Check sheet for the modelled part. Datum: model origin and axes. Units: mm. A direction names the side the tool comes from. Give positions to 0.01 mm unless a question says otherwise; leave off trailing zeros.
from build123d import *

# Parameters (mm, degrees)
SKETCH_4_W          = 150
SKETCH_4_H          = 100
EXTRUDE_1_DEPTH     = 19
EXTRUDE_1_TAPER     = 15
SHELL_1_T           = -2
SKETCH_13_R         = 1.5
CUT_EXTRUDE_3_DEPTH = 92.727858519
CUT_EXTRUDE_4_REACH = 94.119
SKETCH_15_R         = 3.5
SKETCH_16_R         = 2.5
CUT_EXTRUDE_5_DEPTH = 153.623831333


with BuildPart() as part:
    # 草图4 → 凸台-拉伸1 (new body)
    with BuildSketch(Plane(origin=(0, 0, 0), x_dir=(1, 0, 0), z_dir=(0, 1, 0))):
        Rectangle(SKETCH_4_W, SKETCH_4_H)
    extrude(amount=EXTRUDE_1_DEPTH, taper=EXTRUDE_1_TAPER)

    # 抽壳1
    shell_1_openings = [part.faces().sort_by_distance(p)[0] for p in [
        (0, 0, 0),
    ]]
    offset(amount=SHELL_1_T, openings=shell_1_openings, kind=Kind.INTERSECTION)

    # 草图13 → 切除-拉伸3 (cut, through all)
    with BuildSketch(Plane.XZ.offset(-17)):
        with Locations(Location((11, 15, 0), (0, 0, 270))):
            Circle(SKETCH_13_R)
        with Locations(Location((-11, 15, 0), (0, 0, 90))):
            Circle(SKETCH_13_R)
        with Locations(Location((11, -15, 0), (0, 0, 90))):
            Circle(SKETCH_13_R)
        with Locations(Location((-11, -15, 0), (0, 0, 270))):
            Circle(SKETCH_13_R)
    extrude(amount=-CUT_EXTRUDE_3_DEPTH, mode=Mode.SUBTRACT)

    # 切除-拉伸4: up to this plane
    cut_extrude_4_end = Plane(origin=(-75, 0, 50), z_dir=(-0.9659258262890681, 0.2588190451025214, 0))
    # 草图15 → 切除-拉伸4 (cut, up to the surface)
    with BuildSketch(Plane(origin=(0, 0, 0), x_dir=(0, 0, -1), z_dir=(1, 0, 0)), mode=Mode.PRIVATE) as cut_extrude_4_sk1:
        with Locations(Location((-35, 9.5, 0), (0, 0, 90))):
            Circle(SKETCH_15_R)
    cut_extrude_4_tool1 = split(extrude(cut_extrude_4_sk1.sketch, amount=-CUT_EXTRUDE_4_REACH, mode=Mode.PRIVATE), bisect_by=cut_extrude_4_end, keep=Keep.BOTH, mode=Mode.PRIVATE)
    add(cut_extrude_4_tool1.solids().sort_by_distance((0, 9.5, 35))[0], mode=Mode.SUBTRACT)
    # 草图15 → 切除-拉伸4 (cut, up to the surface)
    with BuildSketch(Plane(origin=(0, 0, 0), x_dir=(0, 0, -1), z_dir=(1, 0, 0)), mode=Mode.PRIVATE) as cut_extrude_4_sk2:
        with Locations(Location((35, 9.5, 0), (0, 0, 90))):
            Circle(SKETCH_15_R)
    cut_extrude_4_tool2 = split(extrude(cut_extrude_4_sk2.sketch, amount=-CUT_EXTRUDE_4_REACH, mode=Mode.PRIVATE), bisect_by=cut_extrude_4_end, keep=Keep.BOTH, mode=Mode.PRIVATE)
    add(cut_extrude_4_tool2.solids().sort_by_distance((0, 9.5, -35))[0], mode=Mode.SUBTRACT)

    # 草图16 → 切除-拉伸5 (cut, through all)
    with BuildSketch(Plane(origin=(68.044100989, 18.23236191, 0), x_dir=(0, 0, 1), z_dir=(-0.9659258262890681, -0.2588190451025214, 0))):
        with Locations(Location((0, -11.275834931, 0), (0, 0, 270))):
            Circle(SKETCH_16_R)
    extrude(amount=-CUT_EXTRUDE_5_DEPTH, mode=Mode.SUBTRACT)


solid = part.part
1) Depth check by flat-ended pin: pin 1 Ø4 at (x, z) = (60, 25.5) entering from -Y; pin 2 Ø5 at (y, z) = (6.5, 0.5) entering from -X; pin 3 Ø8 at (y, z) = (9.5, 35) entering from -X. Enter the tip coordinate at first touch or a pass-through.
Recorded:
pin 1: stops at y = 17
pin 2: stops at x = -73.93
pin 3: stops at x = -73.53
2) Set-up check for faces 4 (the face through (-2, 19, 0)), 5 (the face through (-2, 17, 0)), 6 (the face through (-71.44, 11.38, -32.05)): record each of +Z, -Z, +X, -X, +Y, -Y from which the full face is reachable in a straight line by a thin tool's end or side.
Recorded:
face 4: +Z, -Z, +X, -X, +Y
face 5: -Y
face 6: -X
3) Material ranges on L1, parallel to X at y = 18.2, z = 15; L2, parallel to X at y = 17.9, z = -15; L3, parallel to Y at x = 20, z = -32.5, recorded low to high.
Recorded:
L1: x = -70.12 to -12.5, -9.5 to 9.5, 12.5 to 70.12
L2: x = -70.2 to -12.5, -9.5 to 9.5, 12.5 to 70.2
L3: y = 17 to 19
4) Section check A-A, the plane x = 11. State how many separate pieces and enclosed holes the cut face has, then the cut area to 3 significant figures.
Recorded:
separate pieces: 3
enclosed holes: 0
area: 239 mm2
5) Draft check along Y on faces 1 (the face through (-71.44, 11.38, 37.95)), 2 (the face through (-1.02, 8.62, 45.62)), 3 (the face through (11.07, 17.99, 16.5)). Enter one of: +Y half, -Y half, draft (parallel to the pull), parting line (faces both ways), or undercut.
Recorded:
face 1: undercut
face 2: -Y half
face 3: draft
